Read the model definition and answer for the solid it produces. Units are mm, in the model's axes. A direction names the side the tool comes from. Give positions to 0.01 mm unless a question says otherwise; leave off trailing zeros. Write each loop counter-clockwise with the first axis right and the second up, starting at its lowest first coordinate (ties: lowest second). Pieces come first, ordered by that corner, then holes. Notation, with made-up numbers: M 16,-35 L 38,-35 A15 ccw 38,-23 Z; hole C -33,66.5 d5. An arc over 180 degrees is marked long. Put each result on its own line as item: value.
from build123d import *

# Parameters (mm, degrees)
F0_R     = 11
F0_R_2   = 5.5
F1_DEPTH = 3
F2_DEPTH = 12
F3_R     = 2


with BuildPart() as f1:
    # F0 (on Top) → F1 (new body)
    with BuildSketch(Plane.XY):
        Circle(F0_R)
        Circle(F0_R_2, mode=Mode.SUBTRACT)
        Circle(F0_R_2)
    extrude(amount=F1_DEPTH)

    # F0 (on Top) → F2 (join)
    with BuildSketch(Plane.XY):
        Circle(F0_R_2)
    extrude(amount=-F2_DEPTH)

    # F3
    f3_edges = [f1.edges().sort_by_distance(p)[0] for p in [
        (-11, 0, 3),
    ]]
    fillet(f3_edges, radius=F3_R)


solid = f1.part
(1) Section D-D on z = 0.5 is taken. Determine the outline of the cut face in (x, y).
Result:
outline: C 0,0 d22
(2) Which of the six approach directions +Z, -Z, +X, -X, +Y, -Y give full straight-line access (tool end or side, diameter ignored) to faces 1 (the face through (-3, 5, 0)), 2 (the face through (0, 0, 3))?
Result:
face 1: -Z
face 2: +Z, +X, -X, +Y, -Y
(3) Straight lines are drawn through the part: line 1 along Z through (x, y) = (-5, -4.5); line 2 along X through (y, z) = (-0.25, -8.5); line 3 along X through (y, z) = (6.75, 1). For each, find the intervals that lie inside material, in ascending order. Write a range as from..to.
Result:
line 1: z = 0..3
line 2: x = -5.49..5.49
line 3: x = -8.69..8.69
(4) Section C-C on z = -10.25 is taken. Determine the outline of the cut face in (x, y), and give its area (3 significant figures).
Result:
outline: C 0,0 d11
area: 95.0 mm²
(5) Given pin 1 Ø8 at (y, z) = (-4, -10) entering from -X; pin 2 Ø3 at (x, z) = (6, -7) entering from -Y; pin 3 Ø3 at (x, z) = (-3, -2.5) entering from +Y; pin 4 Ø3 at (y, z) = (8, -6) entering from +X, each flat-ended and moving along its own axis, determine where each tip first touches the part or whether it passes through.
Result:
pin 1: stops at x = -5.5
pin 2: stops at y = -3.16
pin 3: stops at y = 5.29
pin 4: passes through
(6) Section A-A on y = 0 is taken. Determine the outline of the cut face in (x, z), and give its area (3 significant figures).
Result:
outline: M -11,0 L -5.5,0 L -5.5,-12 L 5.5,-12 L 5.5,0 L 11,0 L 11,1 A2 ccw 9,3 L -9,3 A2 ccw -11,1 Z
area: 196 mm²
